Could you check a few things on this model? Use its own coordinates, in mm. Face numbers are marked on the shaded views. A direction names the side the tool comes from. Give positions to 0.01 mm unless a question says otherwise; leave off trailing zeros. Order: outer loops, then holes, each group sorted by start corner. A loop starts at its lowest first (then second) coordinate and runs counter-clockwise, first axis right, second up. Notation, with made-up numbers: M -28.5,52.5 L -3.5,52.5 A34 ccw -3.5,89.5 Z; hole C -31,36.5 d10. An arc over 180 degrees is marked long. Return JSON: item names as keys, results as strings. Group by question number.
Autodesk Inventor part; units mm, degrees
ref_plane "YZ Plane" through (0, 0, 0) normal (1, 0, 0) x (0, 1, 0)
ref_plane "XZ Plane" through (0, 0, 0) normal (0, 1, 0) x (-1, 0, 0)
ref_plane "XY Plane" through (0, 0, 0) normal (0, 0, 1) x (1, 0, 0)
sketch "Sketch1" plane through (0, 0, 0) normal (0, 1, 0) x (-1, 0, 0)
  line L0 (34.3343, 23.8125) -> (-51.0732, 23.8125)
  line L1 (-51.0732, 23.8125) -> (-51.0732, -39.6875)
  line L2 (-51.0732, -39.6875) -> (34.3343, -39.6875)
  line L3 (34.3343, -39.6875) -> (34.3343, 23.8125)
  point P0 (0, 0)
  dimension "d0" = 63.5
  dimension "d1" = 85.4075
extrude "Extrusion1" add sketch "Sketch1" along normal blind 14.605
sketch "Sketch2" plane through (0, 0, 0) normal (0, -1, 0) x (1, 0, 0)
  line L0 (-34.3343, 23.8125) -> (51.0732, 23.8125)
  line L1 (32.0232, -39.6875) -> (38.3732, -39.6875)
  line L2 (38.3732, -39.6875) -> (38.3732, 23.8125)
  line L3 (38.3732, 23.8125) -> (32.0232, 23.8125)
  line L4 (32.0232, 13.0175) -> (32.0232, -28.8925)
  line L5 (51.0732, 23.8125) -> (51.0732, -39.6875)
  line L6 (22.4982, -39.6875) -> (38.3732, -39.6875)
  line L7 (38.3732, -39.6875) -> (38.3732, -28.8925)
  line L8 (32.0232, -28.8925) -> (22.4982, -28.8925)
  line L9 (22.4982, -28.8925) -> (22.4982, -39.6875)
  line L10 (22.4982, 23.8125) -> (38.3732, 23.8125)
  line L11 (38.3732, 23.8125) -> (38.3732, 13.0175)
  line L12 (32.0232, 13.0175) -> (22.4982, 13.0175)
  line L13 (22.4982, 13.0175) -> (22.4982, 23.8125)
  point P0 (0, 0)
  dimension "d4" = 63.5
  dimension "d5" = 6.35
  dimension "d6" = 12.7
  dimension "d15" = 10.795
  dimension "d16" = 10.795
  dimension "d17" = 15.875
  dimension "d18" = 15.875
extrude "Extrusion3" add sketch "Sketch2" along normal blind 41.91
sketch "Sketch4" plane through (0, 0, 0) normal (0, -1, 0) x (1, 0, 0)
  line L0 (22.4982, -39.6875) -> (-34.3343, -39.6875)
  line L1 (-34.3343, -39.6875) -> (-34.3343, 23.8125)
  line L2 (-34.3343, 23.8125) -> (22.4982, 23.8125)
  point P0 (0, 0)
  point P1 (-21.6343, -26.9875)
  point P2 (-21.6343, 11.1125)
  point P3 (10.1157, 11.1125)
  point P4 (10.1157, -26.9875)
  dimension "d21" = 12.7
  dimension "d22" = 12.7
  dimension "d23" = 12.7
  dimension "d24" = 12.7
  dimension "d25" = 12.7
  dimension "d26" = 12.7
  dimension "d27" = 44.45
  dimension "d28" = 44.45
hole "Hole1" at (-21.6343, 0, -26.9875) at (-21.6343, 0, 11.1125) at (10.1157, 0, 11.1125) at (10.1157, 0, -26.9875) direction (0, 1, 0) diameter 6.35 end through all
sketch "Sketch5" plane through (0, 0, 0) normal (0, -1, 0) x (1, 0, 0)
  line L0 (38.3732, -39.6875) -> (38.3732, 23.8125)
  line L1 (51.0732, 23.8125) -> (51.0732, -39.6875)
  line L2 (38.3732, 23.8125) -> (51.0732, 23.8125)
  point P0 (0, 0)
  point P1 (44.7232, -7.9375)
  dimension "d36" = 6.35
  dimension "d38" = 31.75
hole "Hole2" at (44.7232, 0, -7.9375) direction (0, 1, 0) diameter 6.35 end through all
properties part number "Vertical sedder motor spacer"
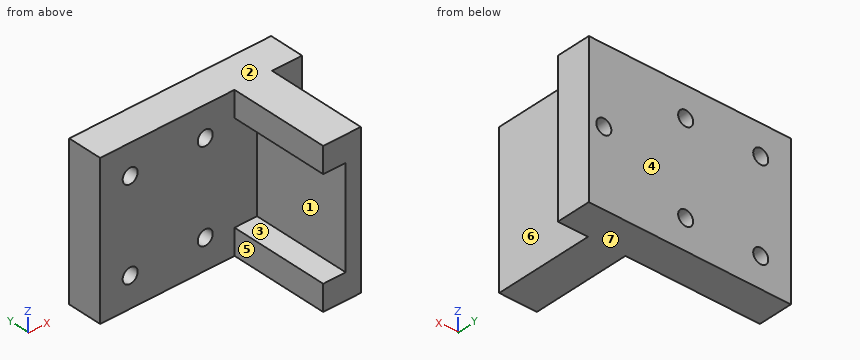
1. Imagine slicing it at C-C, the plane z = -0.5. Please give me the cut outline in (x, y) (3 decimals), plus the area to 3 significant figures.
2. If we mould it in two halves opening along Z, with no side actions, what happens to the marked faces 1, 2, 3 and 4? For each: pulls with the +Z half, pulls with the -Z half, needs draft (parallel to the pull), parting line crosses it, or undercut.
3. Imagine slicing it at D-D, the plane y = 4.5. Count the separate pieces of the cut face and the enclosed holes in it, plus the area to 3 significant figures.
4. Which directions (+Z, -Z, +X, -X, +Y, -Y) give clear straight access to the entire face, cutting with the end or side of a thin tool? Please do the marked faces 5, 6 and 7.
5. For pin 1 (7.5 mm diameter, centred on x = -21.63, z = -26.99, fed in from -Y); pin 2 (3 mm diameter, centred on y = -24, z = -35.5, fed in from -X); pin 3 (10 mm diameter, centred on y = -32.5, z = 3.5, fed in from -X), each with a flat end and sliding along its axis, tell me the tip position at first contact or that it passes through.
6. Imagine slicing it at B-B, the plane x = 8. Please give me the cut outline in (y, z) (1 decimal), plus the area to 3 significant figures.
7. I need wall thicknesses on L1, parallel to Z at x = 28.5, y = -13.5; L2, parallel to X at y = -2, z = -30; L3, parallel to X at y = -21.5, z = -20.5. Which ranges of each line are inside material? Lowest first, please. Write a range as from..to.
8. Imagine slicing it at A-A, the plane z = -8. Please give me the cut outline in (x, y) (3 decimals), plus the area to 3 significant figures.
Values:
{
 "1": {"outline": "M -34.334,0 L 32.023,0 L 32.023,-41.91 L 38.373,-41.91 L 38.373,0 L 51.073,0 L 51.073,14.605 L -34.334,14.605 Z", "area": "1,510 mm²"},
 "2": {"face 1": "undercut", "face 2": "pulls with the +Z half", "face 3": "undercut", "face 4": "needs draft"},
 "3": {"separate pieces": "1", "enclosed holes": "5", "area": "5,270 mm²"},
 "4": {"face 5": "+Z, -Z, -X, -Y", "face 6": "+Z, -Z, +X, -Y", "face 7": "-Z, +X, -X, +Y, -Y"},
 "5": {"pin 1": "stops at y = 0", "pin 2": "stops at x = 22.5", "pin 3": "stops at x = 32.02"},
 "6": {"outline": "M 0,-39.7 L 14.6,-39.7 L 14.6,-29.4 L 0,-29.4 Z; M 0,-24.6 L 14.6,-24.6 L 14.6,8.7 L 0,8.7 Z; M 0,13.5 L 14.6,13.5 L 14.6,23.8 L 0,23.8 Z", "area": "789 mm²"},
 "7": {"L1": "z = -39.69..-28.89, 13.02..23.81", "L2": "x = 22.5..38.37", "L3": "x = 32.02..38.37"},
 "8": {"outline": "M -34.334,0 L 32.023,0 L 32.023,-41.91 L 38.373,-41.91 L 38.373,0 L 41.549,0 L 41.549,14.605 L -34.334,14.605 Z; M 47.898,0 L 51.073,0 L 51.073,14.605 L 47.898,14.605 Z", "area": "1,420 mm²"}
}
